Autodesk Inventor part; units mm, degrees
ref_plane "YZ Plane" through (0, 0, 0) normal (1, 0, 0) x (0, 1, 0)
ref_plane "XZ Plane" through (0, 0, 0) normal (0, 1, 0) x (-1, 0, 0)
ref_plane "XY Plane" through (0, 0, 0) normal (0, 0, 1) x (1, 0, 0)
sketch "Sketch1" plane through (0, 0, 0) normal (0, 0, 1) x (1, 0, 0)
  line L0 (0, 0) -> (25.4, 0)
  line L1 (25.4, 0) -> (25.4, 12.7)
  line L2 (25.4, 12.7) -> (0, 12.7)
  line L3 (0, 12.7) -> (0, 0)
  circle A0 centre (5.08, 6.35) radius 1.5875
  circle A1 centre (17.78, 6.35) radius 1.5875
  dimension "d0" = 12.7
  dimension "d1" = 25.4
  dimension "d2" = 3.175
  dimension "d3" = 3.175
  dimension "d4" = 6.35
  dimension "d5" = 5.08
  dimension "d6" = 12.7
extrude "Extrusion1" add sketch "Sketch1" along normal blind 1.27
sketch "Sketch2" plane through (0, 0, 1.27) normal (0, 0, 1) x (1, 0, 0)
  line L0 (25.4, 12.7) -> (0, 12.7)
  line L1 (25.4, 0) -> (24.13, 0)
  line L2 (24.13, 0) -> (24.13, 12.7)
  line L3 (24.13, 12.7) -> (25.4, 12.7)
  line L4 (25.4, 12.7) -> (25.4, 0)
  point P0 (0, 0)
  dimension "d9" = 1.27
extrude "Extrusion2" add sketch "Sketch2" along normal blind 34.29
sketch "Sketch3" plane through (24.13, 0, 1.27) normal (-1, 0, 0) x (0, 0, 1)
  line L0 (0, 12.7) -> (0, 0)
  line L1 (0, 12.7) -> (34.29, 12.7)
  arc A0 (17.2142, 8.2614) -> (16.0744, 2.794) centre (12.7, 6.35) ccw
  line L2 (17.6022, 6.35) -> (18.5128, 6.35)
  line L3 (18.5128, 6.35) -> (18.5128, 2.794)
  line L4 (18.5128, 2.794) -> (16.0744, 2.794)
  line L5 (16.0744, 2.794) -> (16.0744, 6.35)
  arc A1 (17.8973, 6.35) -> (17.2142, 8.2614) centre (17.5113, 7.2898) ccw
  point P0 (-1.27, 0)
  point P1 (17.2936, 6.35)
  dimension "d21" = 9.8044
  dimension "d22" = 12.7
  dimension "d23" = 6.35
  dimension "d24" = 3.556
  dimension "d25" = 2.4384
  dimension "d26" = 2.032
  dimension "d27" = 0.9398
  dimension "d28" = 3.556
extrude "Extrusion3" cut sketch "Sketch3" against normal blind 25.4
sketch "Sketch4" plane through (24.13, 0, 1.27) normal (-1, 0, 0) x (0, 0, 1)
  line L0 (34.29, 12.7) -> (29.464, 12.7)
  line L1 (29.464, 12.7) -> (29.464, 0)
  line L2 (29.464, 0) -> (34.29, 0)
  line L3 (34.29, 0) -> (34.29, 12.7)
  arc A0 (17.2142, 8.2614) -> (16.0744, 2.794) centre (12.7, 6.35) ccw
  line L4 (0, 0) -> (34.29, 0)
  point P0 (-1.27, 0)
  point P1 (31.877, 0)
  dimension "d29" = 16.764
extrude "Extrusion4" add sketch "Sketch4" along normal blind 4.826
sketch "Sketch5" plane through (19.304, 0, 1.27) normal (-1, 0, 0) x (0, 0, 1)
  line L0 (34.29, 12.7) -> (29.464, 12.7)
  line L1 (29.464, 12.7) -> (29.464, 0)
  line L2 (29.464, 0) -> (34.29, 0)
  line L3 (34.29, 0) -> (34.29, 12.7)
  point P0 (-1.27, 0)
  point P1 (31.8008, 6.35)
  dimension "d33" = 4.826
  dimension "d35" = 12.7
  dimension "d38" = 6.35
  dimension "d46" = 2.3368
hole "Hole1" at (19.304, 6.35, 33.0708) direction (1, 0, 0) diameter 2.4892 end through all
properties part number "000208"
The model under review builds one solid part; all positions refer to its coordinate system, in mm. A direction names the side the tool comes from. Coordinates: 2 decimals unless noted, no trailing zeros. Write each loop counter-clockwise with the first axis right and the second up, starting at its lowest first coordinate (ties: lowest second). Pieces come first, ordered by that corner, then holes.
1) We need section D-D on y = 2. State the section outline as (x, z) points, then the cut area to 3 significant figures.
2) To check wall thickness, follow probe 1 along Y at (x, z) = (17.78, 0.75); probe 2 along Z at (x, y) = (20.75, 3.75); probe 3 along X at (y, z) = (2.75, 23.5). State the ranges of each line that lie inside material, in increasing order.
3) The part is to be moulded in two halves that separate along X. For faces 1 (the face through (25.4, 6, 21)), 2 (the face through (19.304, 8, 33)), 3 (the face through (22, 6, 30.734)), 4 (the face through (16.194, 6.28, 0.626)), say which applies: pulls with the +X half, pulls with the -X half, needs draft (parallel to the pull), parting line crosses it, or undercut.
4) We need section B-B on x = 5.08. State the section outline as (y, z) points.
5) We need section C-C on y = 11.75. State the section outline as (x, z) points, then the cut area to 3 significant figures.
6) We need section A-A on x = 23.5. State the section outline as (y, z) points, then the cut area to 3 significant figures.
7) Machinability: for faces 5 (the face through (25, 5, 19.783)), 6 (the face through (25, 12.7, 17)), 7 (the face through (24.13, 9, 19)), which of the approach directions +Z, -Z, +X, -X, +Y, -Y give a long, thin tool a straight path to every point of the face, cutting with its end or side? Answer none if there is none.
8) Clearance check with flat-ended pins moving along their axes: pin 1 Ø1.4 at (y, z) = (6, 32.5) entering from -X; pin 2 Ø6.5 at (y, z) = (9, 13.5) entering from -X; pin 3 Ø6.5 at (x, y) = (8, 3.5) entering from +Z. State where each tip first meets the part, or that it passes through.
Answer list:
1. outline: (0, 0) - (25.4, 0) - (25.4, 11.71) - (24.13, 11.71) - (24.13, 1.27) - (0, 1.27) - close; (19.3, 30.73) - (24.13, 30.73) - (24.13, 16.23) - (25.4, 16.23) - (25.4, 35.56) - (19.3, 35.56) - close
1. area: 93.4 mm2
2. probe 1: y = 0 to 4.76, 7.94 to 12.7
2. probe 2: z = 0 to 1.27, 30.73 to 35.56
2. probe 3: x = 24.13 to 25.4
3. face 1: pulls with the +X half
3. face 2: pulls with the -X half
3. face 3: needs draft
3. face 4: undercut
4. outline: (0, 0) - (4.76, 0) - (4.76, 1.27) - (0, 1.27) - close; (7.94, 0) - (12.7, 0) - (12.7, 1.27) - (7.94, 1.27) - close
5. outline: (0, 0) - (25.4, 0) - (25.4, 35.56) - (19.3, 35.56) - (19.3, 30.73) - (24.13, 30.73) - (24.13, 1.27) - (0, 1.27) - close
5. area: 99.1 mm2
6. outline: (0, 0) - (12.7, 0) - (12.7, 1.27) - (0, 1.27) - close; (0, 30.73) - (12.7, 30.73) - (12.7, 35.56) - (0, 35.56) - close; hole circle Ø2.49 at (6.35, 33.07)
6. area: 72.6 mm2
7. face 5: +X, -X
7. face 6: +Z, -Z, +X, -X, +Y
7. face 7: -X, +Y, -Y
8. pin 1: stops at x = 19.3
8. pin 2: stops at x = 24.13
8. pin 3: stops at z = 1.27
